```python
from build123d import *

# Parameters (mm, degrees)
F0_W     = 50
F0_H     = 50
F0_W_2   = 40
F0_H_2   = 40
F1_DEPTH = 3
F2_D     = 3
F3_DEPTH = 20
F5_D     = 3
F7_DEPTH = 25


with BuildPart() as f1:
    # F0 (on Top) → F1 (new body)
    with BuildSketch(Plane.XY):
        Rectangle(F0_W, F0_H)
        Rectangle(F0_W_2, F0_H_2, mode=Mode.SUBTRACT)
        Rectangle(F0_W_2, F0_H_2)
    extrude(amount=F1_DEPTH)

    # F2 (through all)
    with Locations(Plane(origin=(0, 0, 0), x_dir=(1, 0, 0), z_dir=(0, 0, -1))):
        with Locations((-20, 20), (20, 20), (20, -20), (-20, -20)):
            Hole(F2_D / 2)

    # F3 (add): a face of the model
    f3_faces = [f1.faces().sort_by_distance(p)[0] for p in [
        (0, -25, 1.5),
    ]]
    extrude(f3_faces, amount=F3_DEPTH)

    # F5 (through all)
    with Locations(Plane(origin=(0, 0, 0), x_dir=(1, 0, 0), z_dir=(0, 0, -1))):
        with Locations((14, 35), (-14, 35)):
            Hole(F5_D / 2)

    # F6 (on face) → F7 (cut)
    with BuildSketch(Plane.XY):
        with BuildLine():
            ThreePointArc((0, -20), (14.1421356237, -14.1421356237), (20, 0))
            ThreePointArc((20, 0), (14.142135611, 14.1421356364), (-3.59e-08, 20))
            ThreePointArc((-3.59e-08, 20), (-14.1421356364, 14.142135611), (-20, 0))
            ThreePointArc((-20, 0), (-14.1421356237, -14.1421356237), (0, -20))
        make_face()
    extrude(amount=F7_DEPTH, mode=Mode.SUBTRACT)


solid = f1.part
```
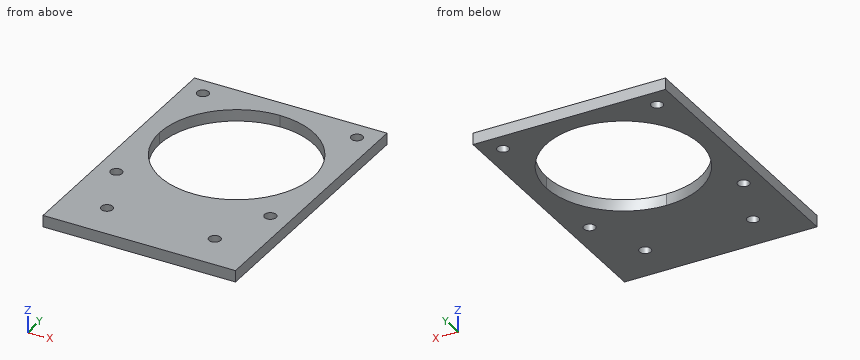
Geometry: final body of the model. Coordinates: model frame, mm. Round coordinates to 2 decimals unless told otherwise and drop trailing zeros. Order: outer loops, then holes, each group sorted by start corner. A loop starts at its lowest first (then second) coordinate and runs counter-clockwise, first axis right, second up. Notation, with made-up numbers: M -2,31.5 L 6,31.5 A18 ccw 6,47.5 Z; hole C 76,88.5 d1. An arc over 180 degrees is marked long. One line per item, written item: value.
(1) Line query: probe 1 along Y at (x, z) = (-14, 2.1); probe 2 along Y at (x, z) = (13.5, 1.95); probe 3 along Y at (x, z) = (0, 0.2). Output: solid intervals per line, ascending. Write a range as [from, to].
Result sheet:
probe 1: [-45, -36.5], [-33.5, -14.28], [14.28, 25]
probe 2: [-45, -36.41], [-33.59, -14.76], [14.76, 25]
probe 3: [-45, -20], [20, 25]
(2) Cut plane D-D (x = -4). Return the cut outline in (y, z).
Result sheet:
outline: M -45,0 L -19.6,0 L -19.6,3 L -45,3 Z; M 19.6,0 L 25,0 L 25,3 L 19.6,3 Z
(3) Pin query (flat end, axial travel): P1, Ø2.5, axis at x = 20, y = -20, coming from the -Z side. Return the tip coordinate at first contact, or that it passes through.
Result sheet:
P1: through
(4) Cut plane A-A (y = 12). Return the cut outline in (x, z).
Result sheet:
outline: M -25,0 L -16,0 L -16,3 L -25,3 Z; M 16,0 L 25,0 L 25,3 L 16,3 Z
(5) Cut plane C-C (x = -14). Return the cut outline in (y, z).
Result sheet:
outline: M -45,0 L -36.5,0 L -36.5,3 L -45,3 Z; M -33.5,0 L -14.28,0 L -14.28,3 L -33.5,3 Z; M 14.28,0 L 25,0 L 25,3 L 14.28,3 Z
(6) Cut plane B-B (z = 1.45). Return the cut outline in (x, y).
Result sheet:
outline: M -25,-45 L 25,-45 L 25,25 L -25,25 Z; hole C -20,-20 d3; hole C -20,20 d3; hole C 0,0 d40; hole C -14,-35 d3; hole C 14,-35 d3; hole C 20,-20 d3; hole C 20,20 d3
